Input: dimensioned drawing with shaded views. Units: mm. Origin: part minimum x, y, z. A direction names the side the tool comes from. Give positions to 0.01 mm unless a question says otherwise; leave off trailing zeros. Write each loop counter-clockwise with the first axis right and the second up, starting at its lowest first coordinate (ties: lowest second). Pieces come first, ordered by that corner, then holes. Notation, with made-up numbers: (26, 61) -> (57, 61) arc R22 cw to (57, 67) -> close; hole circle Ø5 at (75, 36). An arc over 180 degrees is marked (long way). Answer as a JSON object with one key per item and string values.
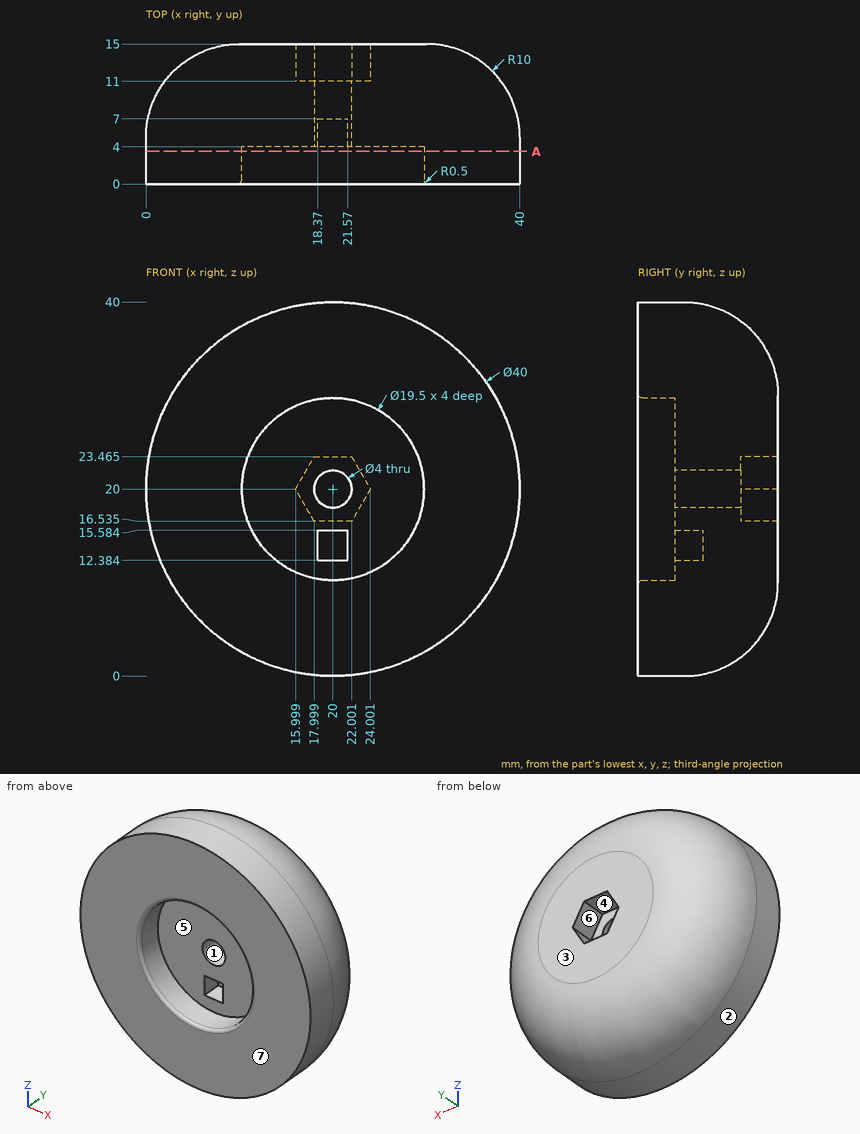
Q1. First-contact query: P1, Ø2, axis at x = 21, y = 12.5, coming from the +Z side; P2, Ø8, axis at x = 30, y = 10, coming from the -Z side; P3, Ø2, axis at x = 20.5, z = 21, coming from the +Y side; P4, Ø3, axis at x = 20, z = 20, coming from the -Y side. Flat tips, straight axial feed; report the tip coordinate or a pass-through.
Values:
{"P1": "z = 37.57", "P2": "z = 1.56", "P3": "y = 11", "P4": "through"}
Q2. Set-up query: the marked faces 5, 6 and 7. Return all of +Z, -Z, +X, -X, +Y, -Y with unobstructed straight access to the full face (end or side cutting, diameter ignored); none if empty.
Values:
{"face 5": "-Y", "face 6": "+Y", "face 7": "+Z, -Z, +X, -X, -Y"}
Q3. Cut plane A-A (y = 3.5). Return the cut outline in (x, z), and give its area (3 significant figures).
Values:
{"outline": "circle Ø40 at (20, 20); hole circle Ø19.5 at (20, 20)", "area": "958 mm²"}
Q4. Mould query, pull axis X, two halves, no side actions, for the marked faces 1, 2, 3 and 4. Classes: pulls with the +X half, pulls with the -X half, needs draft (parallel to the pull), parting line crosses it, or undercut.
Values:
{"face 1": "undercut", "face 2": "parting line crosses it", "face 3": "needs draft", "face 4": "undercut"}
Q5. Material intervals for L1, parallel to Z at x = 20, y = 6.25; L2, parallel to Y at x = 23.5, z = 23.5; L3, parallel to X at y = 0.5, z = 18, sorted ascending. Write a range as from..to.
Values:
{"L1": "0.08..12.38, 15.58..18, 22..39.92", "L2": "4..15", "L3": "0.1..10.46, 29.54..39.9"}
